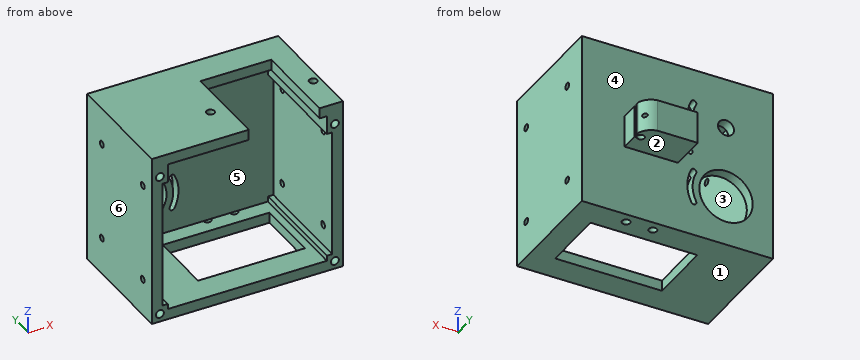
```python
from build123d import *

# Parameters (mm, degrees)
SKETCH1_W                = 64
SKETCH1_H                = 50
BOSS_EXTRUDE1_DEPTH      = 4
SKETCH3_R                = 6.5
CUT_EXTRUDE2_DEPTH       = 4
SKETCH4_W                = 20
SKETCH4_H                = 12
BOSS_EXTRUDE2_DEPTH      = 13.5
CUT_EXTRUDE3_DEPTH       = 47.984039843
CUT_EXTRUDE3_DEPTH_BACK  = 47.984039843
CUT_EXTRUDE4_DEPTH       = 47.984039843
CUT_EXTRUDE4_DEPTH_BACK  = 47.984039843
CUT_EXTRUDE5_DEPTH       = 57.588426379
CUT_EXTRUDE5_DEPTH_BACK  = 57.588426379
SKETCH7_R                = 0.75
CUT_EXTRUDE6_DEPTH       = 54.584046158
CUT_EXTRUDE6_DEPTH_BACK  = 54.584046158
SKETCH8_R                = 1
CUT_EXTRUDE7_DEPTH       = 54.584046158
CUT_EXTRUDE7_DEPTH_BACK  = 54.584046158
SKETCH10_R               = 3
CUT_EXTRUDE8_DEPTH       = 54.584046158
CUT_EXTRUDE8_DEPTH_BACK  = 54.584046158
SKETCH12_W               = 64
SKETCH12_H               = 5
BOSS_EXTRUDE3_DEPTH      = 4
BOSS_EXTRUDE4_DEPTH      = 4
BOSS_EXTRUDE5_DEPTH      = 40.2
SKETCH17_W               = 26.5
SKETCH17_H               = 4
BOSS_EXTRUDE7_DEPTH      = 7.25
SKETCH19_W               = 2
SKETCH19_H               = 7
SKETCH19_H_2             = 2
BOSS_EXTRUDE8_DEPTH      = 40.2
CUT_EXTRUDE9_DEPTH       = 86.529836515
CUT_EXTRUDE9_DEPTH_BACK  = 4
SKETCH18_R               = 1.5
CUT_EXTRUDE10_DEPTH      = 86.599046003
CUT_EXTRUDE10_DEPTH_BACK = 4
SKETCH20_R               = 1.5
SKETCH21_R               = 1.5
CUT_EXTRUDE11_DEPTH      = 4
CUT_EXTRUDE12_DEPTH      = 97.099435462
CUT_EXTRUDE12_DEPTH_BACK = 97.099435462
SKETCH22_R               = 1.25
SKETCH15_W               = 40
SKETCH15_H               = 24.2
CUT_EXTRUDE13_DEPTH      = 10
SKETCH23_R               = 10
CUT_EXTRUDE14_DEPTH      = 78.069468162


with BuildPart() as part:
    # Sketch1 → Boss-Extrude1 (new body)
    with BuildSketch(Plane(origin=(0, 0, 0), x_dir=(1, 0, 0), z_dir=(0, 1, 0))):
        with Locations((1, 15)):
            Rectangle(SKETCH1_W, SKETCH1_H)
    extrude(amount=BOSS_EXTRUDE1_DEPTH)

    # Sketch3 → Cut-Extrude2 (cut)
    with BuildSketch(Plane(origin=(0, 4, 0), x_dir=(1, 0, 0), z_dir=(0, 1, 0))):
        with Locations(Location((-21, 31, 0), (0, 0, 270))):
            Circle(SKETCH3_R)
    extrude(amount=-CUT_EXTRUDE2_DEPTH, mode=Mode.SUBTRACT)

    # Sketch4 → Boss-Extrude2 (add)
    with BuildSketch(Plane(origin=(0, 4, 0), x_dir=(1, 0, 0), z_dir=(0, 1, 0))):
        with Locations((7, 17.5)):
            Rectangle(SKETCH4_W, SKETCH4_H)
    extrude(amount=BOSS_EXTRUDE2_DEPTH)

    # Sketch5 → Cut-Extrude3 (cut, two sides: drawn at the far end of the back side and taken through both)
    with BuildSketch(Plane.XY.offset(-11.5).offset(-CUT_EXTRUDE3_DEPTH_BACK)):
        with BuildLine():
            Line((17, 10.75), (16.152443057, 10.75))
            ThreePointArc((16.152443057, 10.75), (13.625, 11.5), (16.152443057, 12.25))
            Line((16.152443057, 12.25), (19, 12.25))
            Line((19, 12.25), (22.19672231, 12.25))
            Line((22.19672231, 12.25), (22.19672231, 10.75))
            Line((22.19672231, 10.75), (17, 10.75))
        make_face()
    extrude(amount=CUT_EXTRUDE3_DEPTH + CUT_EXTRUDE3_DEPTH_BACK, mode=Mode.SUBTRACT)

    # Sketch6 → Cut-Extrude4 (cut, two sides: drawn at the far end of the back side and taken through both)
    with BuildSketch(Plane.XY.offset(-11.5).offset(-CUT_EXTRUDE4_DEPTH_BACK)):
        with BuildLine():
            Line((12, 17.5), (17, 17.5))
            Line((17, 17.5), (17, 13.25))
            ThreePointArc((17, 13.25), (15.124760231, 16.110012037), (12, 17.5))
        make_face()
    extrude(amount=CUT_EXTRUDE4_DEPTH + CUT_EXTRUDE4_DEPTH_BACK, mode=Mode.SUBTRACT)

    # Sketch7 → Cut-Extrude5 (cut, two sides: drawn at the far end of the back side and taken through both)
    with BuildSketch(Plane.ZY.offset(3).offset(-CUT_EXTRUDE5_DEPTH_BACK)):
        with Locations((-17.5, 15.5)):
            Circle(SKETCH7_R)
    extrude(amount=CUT_EXTRUDE5_DEPTH + CUT_EXTRUDE5_DEPTH_BACK, mode=Mode.SUBTRACT)

    # Sketch8 → Cut-Extrude6 (cut, two sides: drawn at the far end of the back side and taken through both)
    with BuildSketch(Plane(origin=(0, 4, 0), x_dir=(1, 0, 0), z_dir=(0, 1, 0)).offset(-CUT_EXTRUDE6_DEPTH_BACK)):
        with Locations(Location((-7.5, 31, 0), (0, 0, 270))):
            Circle(SKETCH8_R)
        with Locations(Location((-7.5, 17.5, 0), (0, 0, 270))):
            Circle(SKETCH8_R)
        with Locations(Location((-7.5, 4, 0), (0, 0, 270))):
            Circle(SKETCH8_R)
    extrude(amount=CUT_EXTRUDE6_DEPTH + CUT_EXTRUDE6_DEPTH_BACK, mode=Mode.SUBTRACT)

    # Sketch10 → Cut-Extrude7 (cut, two sides: drawn at the far end of the back side and taken through both)
    with BuildSketch(Plane(origin=(0, 4, 0), x_dir=(1, 0, 0), z_dir=(0, 1, 0)).offset(-CUT_EXTRUDE7_DEPTH_BACK)):
        with Locations(Location((-21, 4, 0), (0, 0, 270))):
            Circle(SKETCH10_R)
    extrude(amount=CUT_EXTRUDE7_DEPTH + CUT_EXTRUDE7_DEPTH_BACK, mode=Mode.SUBTRACT)

    # Sketch11 → Cut-Extrude8 (cut, two sides: drawn at the far end of the back side and taken through both)
    with BuildSketch(Plane(origin=(0, 4, 0), x_dir=(1, 0, 0), z_dir=(0, 1, 0)).offset(-CUT_EXTRUDE8_DEPTH_BACK)):
        with BuildLine():
            ThreePointArc((-9.802419794, 25.444444444), (-8.5, 31), (-9.802419794, 36.555555556))
            ThreePointArc((-9.802419794, 36.555555556), (-9.351057822, 37.895806416), (-8.010806961, 37.444444444))
            ThreePointArc((-8.010806961, 37.444444444), (-6.5, 31), (-8.010806961, 24.555555556))
            ThreePointArc((-8.010806961, 24.555555556), (-9.351057822, 24.104193584), (-9.802419794, 25.444444444))
        make_face()
        with BuildLine():
            ThreePointArc((-9.802419794, 9.555555556), (-8.5, 4), (-9.802419794, -1.555555556))
            ThreePointArc((-9.802419794, -1.555555556), (-9.351057822, -2.895806416), (-8.010806961, -2.444444444))
            ThreePointArc((-8.010806961, -2.444444444), (-6.5, 4), (-8.010806961, 10.444444444))
            ThreePointArc((-8.010806961, 10.444444444), (-9.351057822, 10.895806416), (-9.802419794, 9.555555556))
        make_face()
    extrude(amount=CUT_EXTRUDE8_DEPTH + CUT_EXTRUDE8_DEPTH_BACK, mode=Mode.SUBTRACT)

    # Sketch12 → Boss-Extrude3 (add)
    with BuildSketch(Plane(origin=(0, 4, 0), x_dir=(1, 0, 0), z_dir=(0, 1, 0))):
        with Locations((1, 42.5)):
            Rectangle(SKETCH12_W, SKETCH12_H)
        with Locations((1, -12.5)):
            Rectangle(SKETCH12_W, SKETCH12_H)
    extrude(amount=-BOSS_EXTRUDE3_DEPTH)

    # Sketch13 → Boss-Extrude4 (add)
    with BuildSketch(Plane(origin=(0, 0, 0), x_dir=(1, 0, 0), z_dir=(0, 1, 0))):
        Polygon((33, 38.853125133), (-31, 38.853125133), (-31, -15), (-38.545432929, -15), (-38.545432929, 50.003125133), (-31, 50.003125133), (33, 50.003125133), align=None)
    extrude(amount=BOSS_EXTRUDE4_DEPTH)

    # Sketch14 → Boss-Extrude5 (add)
    with BuildSketch(Plane.XZ):
        Polygon((-38.545432929, 15), (-2.245432929, 15), (-2.245432929, 11), (-34.545432929, 11), (-34.545432929, -46.003125133), (29, -46.003125133), (29, 11), (24.254567071, 11), (24.254567071, 15), (33, 15), (33, 4.2), (33, -50.003125133), (29, -50.003125133), (-34.545432929, -50.003125133), (-38.545432929, -50.003125133), (-38.545432929, 4.2), align=None)
    extrude(amount=BOSS_EXTRUDE5_DEPTH)

    # Sketch17 → Boss-Extrude7 (add)
    with BuildSketch(Plane.XZ):
        with Locations((11.004567071, 13)):
            Rectangle(SKETCH17_W, SKETCH17_H)
    extrude(amount=BOSS_EXTRUDE7_DEPTH)

    # Sketch19 → Boss-Extrude8 (add)
    with BuildSketch(Plane.XZ.offset(40.2)):
        with Locations((-33.545432929, 7.5)):
            Rectangle(SKETCH19_W, SKETCH19_H)
        with Locations((-33.545432929, -45.003125133)):
            Rectangle(SKETCH19_W, SKETCH19_H_2)
        with Locations((28, -45.003125133)):
            Rectangle(SKETCH19_W, SKETCH19_H_2)
        with Locations((28, 7.5)):
            Rectangle(SKETCH19_W, SKETCH19_H)
    extrude(amount=-BOSS_EXTRUDE8_DEPTH)

    # Sketch18 → Cut-Extrude9 (cut, two sides: drawn at the far end of the back side and taken through both)
    with BuildSketch(Plane.XZ.offset(40.2).offset(-CUT_EXTRUDE9_DEPTH_BACK)):
        with Locations(Location((-35.545432929, 7, 0), (0, 0, 90))):
            Circle(SKETCH18_R)
        with Locations(Location((30, 7, 0), (0, 0, 90))):
            Circle(SKETCH18_R)
        with Locations(Location((30, -47.003125133, 0), (0, 0, 90))):
            Circle(SKETCH18_R)
        with Locations(Location((-35.545432929, -47.003125133, 0), (0, 0, 90))):
            Circle(SKETCH18_R)
    extrude(amount=CUT_EXTRUDE9_DEPTH + CUT_EXTRUDE9_DEPTH_BACK, mode=Mode.SUBTRACT)

    # Sketch20 → Cut-Extrude10 (cut, two sides: drawn at the far end of the back side and taken through both)
    with BuildSketch(Plane.XY.offset(15).offset(-CUT_EXTRUDE10_DEPTH_BACK)):
        with Locations(Location((-8.245432929, -24.95, 0), (0, 0, 180))):
            Circle(SKETCH20_R)
        with Locations(Location((30.254567071, -24.95, 0), (0, 0, 180))):
            Circle(SKETCH20_R)
    extrude(amount=CUT_EXTRUDE10_DEPTH + CUT_EXTRUDE10_DEPTH_BACK, mode=Mode.SUBTRACT)

    # Sketch21 → Cut-Extrude11 (cut)
    with BuildSketch(Plane(origin=(0, 0, -50.003125133), x_dir=(-1, 0, 0), z_dir=(0, 0, -1))):
        with Locations((-4.227283535, 0)):
            Circle(SKETCH21_R)
        with Locations((-14.227283535, 0)):
            Circle(SKETCH21_R)
    extrude(amount=-CUT_EXTRUDE11_DEPTH, mode=Mode.SUBTRACT)

    # Sketch22 → Cut-Extrude12 (cut, two sides: drawn at the far end of the back side and taken through both)
    with BuildSketch(Plane(origin=(33, 0, 0), x_dir=(0, 0, -1), z_dir=(1, 0, 0)).offset(-CUT_EXTRUDE12_DEPTH_BACK)):
        with Locations((-1, -6)):
            Circle(SKETCH22_R)
        with Locations((36, -34)):
            Circle(SKETCH22_R)
        with Locations((-1, -34)):
            Circle(SKETCH22_R)
        with Locations((36, -6)):
            Circle(SKETCH22_R)
    extrude(amount=CUT_EXTRUDE12_DEPTH + CUT_EXTRUDE12_DEPTH_BACK, mode=Mode.SUBTRACT)

    # Sketch15 → Cut-Extrude13 (cut)
    with BuildSketch(Plane.XY.offset(-46.003125133)):
        with Locations((4.254567071, -18.1)):
            Rectangle(SKETCH15_W, SKETCH15_H)
    extrude(amount=-CUT_EXTRUDE13_DEPTH, mode=Mode.SUBTRACT)

    # Sketch23 → Cut-Extrude14 (cut, through all)
    with BuildSketch(Plane(origin=(0, 4, 0), x_dir=(1, 0, 0), z_dir=(0, 1, 0))):
        with Locations(Location((-21, 31, 0), (0, 0, 270))):
            Circle(SKETCH23_R)
    extrude(amount=-CUT_EXTRUDE14_DEPTH, mode=Mode.SUBTRACT)


solid = part.part
```
Geometry check sheet. Reference: the model listing, model coordinates, mm. Face numbers are marked on the shaded views. A direction names the side the tool comes from. Coordinates: 2 decimals unless noted, no trailing zeros. Write each loop counter-clockwise with the first axis right and the second up, starting at its lowest first coordinate (ties: lowest second). Pieces come first, ordered by that corner, then holes. Notation, with made-up numbers: M -34.75,68 L 19.25,68 A29 cw 19.25,101 Z; hole C 29,87 d11. An arc over 180 degrees is marked long. One line per item, written item: value. Start each with the question number.
(1) Sectioned sample at B-B, the plane x = 21. Enter the section's corners in (y, z).
(2) Tool access check on the marked faces 1, 2 and 3. Record the directions out of +Z, -Z, +X, -X, +Y, -Y that give a thin tool (end or side, any length) a straight path to the whole face; none if there is none.
(3) Sectioned sample at A-A, the plane z = -4. Enter the section's corners in (x, y).
(4) Release check for a two-part mould opening along X. For the marked faces 4, 5 and 6 record: released by +X, released by -X, zero draft, split by the parting line, or undercut.
(5) Scan lines: line 1 along X through (y, z) = (1.75, -4); line 2 along Y through (x, z) = (-36.95, -36); line 3 along X through (y, z) = (1, -31). Record each from-to range of solid material in increasing order. Write a range as [from, to].
(6) Depth check by flat-ended pin: pin 1 (13 mm diameter, centred on y = 8, z = -16, fed in from -X); pin 2 (8 mm diameter, centred on x = -21, z = -4, fed in from -Y); pin 3 (12 mm diameter, centred on x = 13, z = 6, fed in from -Y); pin 4 (5.5 mm diameter, centred on y = 7, z = -20.5, fed in from +X). Enter the tip coordinate at first touch or a pass-through.
(7) Sectioned sample at C-C, the plane x = -21. Enter the section's corners in (y, z), and give its area (3 significant figures).
Filled sheet:
1. outline: M -40.2,-50 L -30.2,-50 L -30.2,-46 L -40.2,-46 Z; M -7.25,11 L 0,11 L 0,-46 L -6,-46 L -6,-50 L 4,-50 L 4,15 L -7.25,15 Z
2. face 1: -Z, +X, -X, +Y, -Y
2. face 2: -Z, +X, -X, +Y
2. face 3: -Y
3. outline: M -38.55,-40.2 L -34.55,-40.2 L -34.55,0 L -24,0 L -24,4 L -38.55,4 Z; M -18,0 L -8.5,0 L -8.5,4 L -18,4 Z; M -6.5,0 L 29,0 L 29,-40.2 L 33,-40.2 L 33,4 L -6.5,4 Z
4. face 4: zero draft
4. face 5: undercut
4. face 6: released by -X
5. line 1: [-38.55, -24], [-18, -8.5], [-6.5, 33]
5. line 2: [-40.2, -35.25], [-32.75, -7.25], [-4.75, 4]
5. line 3: [-38.55, -31], [-11, -8.5], [-6.5, 33]
6. pin 1: x = -38.55
6. pin 2: y = 0
6. pin 3: y = -7.25
6. pin 4: x = 17
7. outline: M -40.2,-50 L 4,-50 L 4,-41 L 0,-41 L 0,-46 L -40.2,-46 Z; M -40.2,11 L 0,11 L 0,-1 L 4,-1 L 4,15 L -40.2,15 Z; M 0,-21 L 4,-21 L 4,-7 L 0,-7 Z
7. area: 478 mm²
